Verification items for the finished model (mm, model axes). A direction names the side the tool comes from. Give positions to 0.01 mm unless a question says otherwise; leave off trailing zeros. Order: outer loops, then holes, each group sorted by start corner. A loop starts at its lowest first (then second) coordinate and runs counter-clockwise, first axis right, second up. Notation, with made-up numbers: (37, 52.5) -> (76, 52.5) arc R28 ccw to (76, 88.5) -> close; hole circle Ø1 at (43, -37.5). An arc over 180 degrees is marked (long way). Write each question's results on one line, items separated by ' | '. Start each with the question number.
1. Cross-section at C-C, the plane y = 6.75. Enter the section's corners in (x, z).
2. Depth check by flat-ended pin: pin 1 Ø6 at (x, z) = (9.5, 186) entering from +Y; pin 2 Ø2.5 at (y, z) = (5.5, 330) entering from +X. Enter the tip coordinate at first touch or a pass-through.
3. Cross-section at A-A, the plane x = 6.35. Enter the section's corners in (y, z).
4. Set-up check for faces 1 (the face through (7, 0, 250)), 2 (the face through (7, 1.27, 250)): record each of +Z, -Z, +X, -X, +Y, -Y from which the full face is reachable in a straight line by a thin tool's end or side.
5. Material ranges on L1, parallel to Z at x = 6.35, y = 0.3; L2, parallel to X at y = 10.5, z = 327.5, recorded low to high. Write a range as from..to.
Autodesk Inventor part; units mm, degrees
ref_plane "YZ Plane" through (0, 0, 0) normal (1, 0, 0) x (0, 1, 0)
ref_plane "XZ Plane" through (0, 0, 0) normal (0, 1, 0) x (-1, 0, 0)
ref_plane "XY Plane" through (0, 0, 0) normal (0, 0, 1) x (1, 0, 0)
sketch "Sketch1" plane through (0, 0, 0) normal (0, 0, 1) x (1, 0, 0)
  line L0 (0, 0) -> (12.7, 0)
  line L1 (12.7, 0) -> (12.7, 1.27)
  line L2 (12.7, 1.27) -> (1.27, 1.27)
  line L3 (1.27, 1.27) -> (1.27, 12.7)
  line L4 (1.27, 12.7) -> (0, 12.7)
  line L5 (0, 12.7) -> (0, 0)
  dimension "d0" = 12.7
  dimension "d1" = 1.27
  dimension "d2" = 11.43
extrude "Extrusion1" add sketch "Sketch1" along normal blind 508
fillet "Fillet1" radius 1.27 4 edges at (12.7, 1.27, 254) (1.27, 12.7, 254) (1.27, 1.27, 254) (0, 0, 254)
sketch "Sketch2" plane through (2.54, 1.27, 508) normal (0, 1, 0) x (1, 0, 0)
  line L0 (0, 0) -> (0, 508)
  line L1 (8.89, 0) -> (0, 0)
  line L2 (8.89, 508) -> (8.89, 0)
  circle A0 centre (3.81, 6.35) radius 2.4892
  line L3 (-2.54, 0) -> (-2.54, 508)
  line L4 (-2.54, 508) -> (-2.54, 0)
  line L5 (8.89, 254) -> (0, 254) construction
  circle A1 centre (3.81, 501.65) radius 2.4892
  dimension "d6" = 4.9784
  dimension "d7" = 6.35
  dimension "d8" = 6.35
extrude "Extrusion2" cut sketch "Sketch2" against normal blind 25.4
properties part number ".05 in Aluminum Angle" material "Aluminum 6061"
Results below:
1) outline: (0, 0) -> (1.27, 0) -> (1.27, 508) -> (0, 508) -> close
2) pin 1: stops at y = 1.27 | pin 2: stops at x = 1.27
3) outline: (0, 0) -> (1.27, 0) -> (1.27, 3.86) -> (0, 3.86) -> close; (0, 8.84) -> (1.27, 8.84) -> (1.27, 499.16) -> (0, 499.16) -> close; (0, 504.14) -> (1.27, 504.14) -> (1.27, 508) -> (0, 508) -> close
4) face 1: +Z, -Z, +X, -X, -Y | face 2: +Z, -Z, +X, +Y
5) L1: z = 0..3.86, 8.84..499.16, 504.14..508 | L2: x = 0..1.27
